Design review of the part built by this model. Coordinates are the model's own, in mm. A direction names the side the tool comes from. Round coordinates to 2 decimals unless told otherwise and drop trailing zeros. Write each loop counter-clockwise with the first axis right and the second up, starting at its lowest first coordinate (ties: lowest second). Pieces come first, ordered by that corner, then holes. Notation, with made-up numbers: (-2.75, 58.5) - (24.25, 58.5) arc R18 cw to (24.25, 71.5) - close; hole circle Ø4 at (42, -19.75). An arc over 180 degrees is marked (long way). Use one line per item in the form item = value.
```python
from build123d import *

# Parameters (mm, degrees)
SKETCH_2_W          = 5
SKETCH_2_H          = 5
SKETCH_2_W_2        = 10
SKETCH_2_H_2        = 15
EXTRUDE_1_DEPTH     = 20
FILLET_1_R          = 10
FILLET_2_R          = 5
SKETCH_3_R          = 5
CUT_EXTRUDE_1_DEPTH = 38.749172176


with BuildPart() as part:
    # 草圖2 → 填料-伸長1 (new body)
    with BuildSketch(Plane.XY):
        with Locations((2.5, -2.5)):
            Rectangle(SKETCH_2_W, SKETCH_2_H)
        with Locations((10, -2.5)):
            Rectangle(SKETCH_2_W_2, SKETCH_2_H)
        with Locations((2.5, -12.5)):
            Rectangle(SKETCH_2_W, SKETCH_2_H_2)
        Polygon((5, -20), (0, -20), (0, -25), (25, -25), (25, -20), align=None)
    extrude(amount=-EXTRUDE_1_DEPTH)

    # 圓角1
    fillet_1_edges = [part.edges().sort_by_distance(p)[0] for p in [
        (25, -22.5, 0),
        (25, -22.5, -20),
        (0, -25, -10),
    ]]
    fillet(fillet_1_edges, radius=FILLET_1_R - 0.0001)  # a hair under: the kernel refuses the full size

    # 圓角2
    fillet_2_edges = [part.edges().sort_by_distance(p)[0] for p in [
        (15, -2.5, -20),
        (15, -2.5, 0),
        (5, -20, -10),
    ]]
    fillet(fillet_2_edges, radius=FILLET_2_R)

    # 草圖3 → 除料-伸長1 (cut, through all)
    with BuildSketch(Plane(origin=(0, -20, 0), x_dir=(1, 0, 0), z_dir=(0, 1, 0))):
        with Locations(Location((15, 10, 0), (0, 0, 180))):
            Circle(SKETCH_3_R)
    extrude(amount=-CUT_EXTRUDE_1_DEPTH, mode=Mode.SUBTRACT)


solid = part.part
```
Q1. Machinability: for faces 1 (the flat face through (21, -20, -10)), 2 (the cylindrical face through (13, -2, -19)), 3 (the cylindrical face through (13, -2, -1)), 4 (the cylindrical face through (19, -22, -7)), 5 (the cylindrical face through (2.85, -21.99, -10.14)), which of the approach directions +Z, -Z, +X, -X, +Y, -Y give a long, thin tool a straight path to every point of the face, cutting with its end or side? Answer none if there is none.
Calculated:
face_1 = +Z, -Z, +X
face_2 = -Z, +X, +Y
face_3 = +Z, +X, +Y
face_4 = -Y
face_5 = +Z, -Z, -X, -Y
Q2. To check wall thickness, follow line 1 along Z through (x, y) = (15, -22.75); line 2 along Y through (x, z) = (12.5, -4.75); line 3 along X through (y, z) = (-7.25, -8). State the ranges of each line that lie inside material, in increasing order. Write a range as from..to.
Calculated:
line_1 = -20..-15, -5..0
line_2 = -25..-20, -5..0
line_3 = 0..5
Q3. For P1, Ø3, axis at x = 7.5, z = -9.5, coming from the -Y side; P2, Ø4, axis at y = -2, z = -12, coming from the +X side; P3, Ø6, axis at y = -10.5, z = -5, coming from the +X side, all flat-tipped, find the tip position at first contact; note any pin that passes through.
Calculated:
P1 = -24.95
P2 = 15
P3 = 5
Q4. We need section C-C on x = 6.25. Write out the cut boundary in (y, z).
Calculated:
outline = (-24.27, -20) - (-18.31, -20) - (-18.31, 0) - (-24.27, 0) - close; (-5, -20) - (0, -20) - (0, 0) - (-5, 0) - close
Q5. Draft analysis for pull direction Y (two halves, no side actions). For faces 6 (the flat face through (8, 0, -10)), 7 (the flat face through (4, -12, 0)), 8 (the cylindrical face through (7, -19, -10)), 9 (the flat face through (5, -10, -10)), state which applies: released by +Y, released by -Y, zero draft, split by the parting line, or undercut.
Calculated:
face_6 = released by +Y
face_7 = zero draft
face_8 = undercut
face_9 = undercut
Q6. We need section D-D on z = -17.5. Write out the cut boundary in (x, y).
Calculated:
outline = (0, -15) arc R10 ccw to (10, -25) - (21.61, -25) - (21.61, -20) - (10, -20) arc R5 cw to (5, -15) - (5, -5) - (14.33, -5) - (14.33, 0) - (0, 0) - close
Q7. We need section B-B on x = 12. Write out the cut boundary in (y, z).
Calculated:
outline = (-25, -20) - (-20, -20) - (-20, -14) - (-25, -14) - close; (-25, -6) - (-20, -6) - (-20, 0) - (-25, 0) - close; (-5, -19.58) - (0, -19.58) - (0, -0.42) - (-5, -0.42) - close
